```python
from build123d import *

# Parameters (mm, degrees)
SKETCH3_W = 7.366
SKETCH3_H = 1.5


with BuildPart() as part:
    # Sweep1: sweep along a path in Sketch2
    with BuildLine(Plane.XY) as sweep1_path:
        Line((7.091056719, -457.202005016), (7.218056719, -0.002005016))
        ThreePointArc((7.218056719, -0.002005016), (-0.072338406, 7.217694506), (-7.216566601, -0.146674154))
        Line((-7.216566601, -0.146674154), (-0.57395254, -326.972262728))
        ThreePointArc((-0.57395254, -326.972262728), (-0.574097453, -341.338325894), (-1.158260966, -355.692507303))
        Line((-1.158260966, -355.692507303), (-7.331629374, -456.759929099))
        ThreePointArc((-7.331629374, -456.759929099), (-0.348139893, -464.414668667), (7.091056719, -457.202005016))
    # Sketch3 → Sweep1 (sweep)
    with BuildSketch(Plane(origin=(0, 0, 0), x_dir=(0, 0, -1), z_dir=(1, 0, 0))):
        with Locations((3.683, 7.887099691)):
            Rectangle(SKETCH3_W, SKETCH3_H)
    sweep(path=sweep1_path.line)


solid = part.part
```
Work out the finished part from the listing and answer in its coordinate system (mm). A direction names the side the tool comes from. Round coordinates to 2 decimals unless told otherwise and drop trailing zeros. Write each loop counter-clockwise with the first axis right and the second up, starting at its lowest first coordinate (ties: lowest second). Pieces come first, ordered by that corner, then holes. Notation, with made-up numbers: (33, -33) -> (42, -33) arc R20 cw to (42, -3) -> close; hole circle Ø2 at (-34.5, -5.75). An arc over 180 degrees is marked (long way). Write each question's results on one line, items separated by ' | '.
1) The part is cut by section A-A (z = -2.75). Write down the section's boundary in (x, y), and give its area (3 significant figures).
Findings:
outline: (-8.75, -456.67) arc R8.64 ccw (long way) to (8.51, -457.2) -> (8.64, 0) arc R8.64 ccw (long way) to (-8.64, -0.18) -> (-1.99, -327) arc R351.89 cw to (-2.57, -355.61) -> close; hole (-7.25, -456.76) arc R7.14 ccw (long way) to (7.01, -457.2) -> (7.14, 0) arc R7.14 ccw (long way) to (-7.14, -0.15) -> (-0.49, -326.97) arc R353.39 cw to (-1.08, -355.7) -> close | area: 1,450 mm²
2) Which of the six approach directions +Z, -Z, +X, -X, +Y, -Y give full straight-line access (tool end or side, diameter ignored) to faces 1 (the flat face through (-4.207, -406.939, -3.631)), 2 (the flat face through (-5.7, -406.8, -3.7)), 3 (the flat face through (-3, -227, 0))?
Findings:
face 1: +Z, -Z | face 2: +Z, -Z, -X | face 3: +Z, +X, -X, +Y, -Y
3) The part is cut by section C-C (x = 3.5). Write down the section's boundary in (y, z), and give its area (3 significant figures).
Findings:
outline: (-465.04, -7.37) -> (-463.35, -7.37) -> (-463.35, 0) -> (-465.04, 0) -> close; (6.22, -7.37) -> (7.9, -7.37) -> (7.9, 0) -> (6.22, 0) -> close | area: 24.8 mm²
4) For a pull along Y with two mould halves and no side action, classify faces 4 (the cylindrical face through (-0.506, -464.327, -3.735)), 5 (the flat face through (-3, -227, -7.366)) as +Y half, -Y half, draft (parallel to the pull), parting line (faces both ways), or undercut.
Findings:
face 4: undercut | face 5: draft
5) Consider line 1 along X through (y, z) = (-70, -1.5); line 2 along X through (y, z) = (-175, -1); line 3 along Y through (x, z) = (4.5, -1.75). Determine where each line is inside the solid, lowest interval first. Write a range as [from, to].
Findings:
line 1: x = [-7.22, -5.72], [7.12, 8.62] | line 2: x = [-5.08, -3.58], [7.09, 8.59] | line 3: y = [-464.49, -462.63], [5.54, 7.37]
6) The part is cut by section B-B (y = -335). Write down the section's boundary in (x, z).
Findings:
outline: (-1.92, -7.37) -> (-0.42, -7.37) -> (-0.42, 0) -> (-1.92, 0) -> close; (7.04, -7.37) -> (8.54, -7.37) -> (8.54, 0) -> (7.04, 0) -> close
7) Flat-ended cylindrical pins translate along their axes: pin 1 (2 mm diameter, centred on x = 3.5, z = -6.5, fed in from -Y); pin 2 (2 mm diameter, centred on x = 6, y = -230.5, fed in from +Z); pin 3 (2 mm diameter, centred on x = 5.5, z = -4.5, fed in from -Y); pin 4 (3 mm diameter, centred on x = 4.5, z = -5, fed in from -Y). Find the tip coordinate at first contact, or state that the pin passes through.
Findings:
pin 1: stops at y = -465.43 | pin 2: passes through | pin 3: stops at y = -464.49 | pin 4: stops at y = -465.25
